For this review, take the finished solid that the model builds, in its own axes (mm). A direction names the side the tool comes from. Give positions to 0.01 mm unless a question says otherwise; leave off trailing zeros. Write each loop counter-clockwise with the first axis right and the second up, starting at its lowest first coordinate (ties: lowest second). Pieces come first, ordered by that corner, then holes. Notation, with made-up numbers: (12.25, 76.25) -> (44.25, 76.25) arc R14 cw to (44.25, 103.25) -> close; hole circle Ø7 at (-34.75, 7). An arc over 180 degrees is marked (long way). Answer as CSV lines item,"result".
```python
from build123d import *

# Parameters (mm, degrees)
BOX001_W           = 93.5
BOX001_H           = 21.5
BOX001_DEPTH       = 20.75
BOX015001015_W     = 96.5
BOX015001015_H     = 24.5
BOX015001015_DEPTH = 22.25


with BuildPart() as cube016:
    # Box001 → Box001 (new body)
    with BuildSketch(Plane(origin=(1.5, 1.5, 1.5), x_dir=(1, 0, 0), z_dir=(0, 0, 1))):
        with Locations((46.75, 10.75)):
            Rectangle(BOX001_W, BOX001_H)
    extrude(amount=BOX001_DEPTH)


with BuildPart() as cut004014:
    # Box015001015 → Box015001015 (new body)
    with BuildSketch(Plane.XY):
        with Locations((48.25, 12.25)):
            Rectangle(BOX015001015_W, BOX015001015_H)
    extrude(amount=BOX015001015_DEPTH)

    # Cut004014: cut Cube016
    add(cube016.part, mode=Mode.SUBTRACT)


with BuildPart() as cut004014_1:
    # Cut004014 placement: moved
    add(cut004014.part.moved(Location((3, -4, 0))))


solid = cut004014_1.part
```
Q1. Clearance check with a flat-ended pin moving along its axis: pin 1 (6.5 mm diameter, centred on x = 40, y = 12, fed in from +Z). State where the tip first meets the part, or that it passes through.
Answer block:
pin 1,"stops at z = 1.5"
Q2. Add section C-C (x = 44.5). Write out the cut boundary in (y, z), plus the area to 3 significant figures.
Answer block:
outline,"(-4, 0) -> (20.5, 0) -> (20.5, 22.25) -> (19, 22.25) -> (19, 1.5) -> (-2.5, 1.5) -> (-2.5, 22.25) -> (-4, 22.25) -> close"
area,"99.0 mm2"
Q3. To check wall thickness, follow probe 1 along X at (y, z) = (16, 1.75); probe 2 along Y at (x, z) = (63.5, 17.5); probe 3 along Z at (x, y) = (35.5, -2.25). State the ranges of each line that lie inside material, in increasing order. Write a range as [from, to].
Answer block:
probe 1,"x = [3, 4.5], [98, 99.5]"
probe 2,"y = [-4, -2.5], [19, 20.5]"
probe 3,"z = [0, 1.5]"
Q4. For faces 4 (the flat face through (51, 8, 1.5)), 5 (the flat face through (99.5, 8, 11)), list the 3-axis set-ups (+Z, -Z, +X, -X, +Y, -Y) from which the entire face can be reached by the end or side of a thin tool; tool diameter is ignored.
Answer block:
face 4,"+Z"
face 5,"+Z, -Z, +X, +Y, -Y"
Q5. Draft analysis for pull direction X (two halves, no side actions). For faces 1 (the flat face through (3, 8, 11)), 2 (the flat face through (51, 8, 0)), 3 (the flat face through (51, 19, 12)), state which applies: released by +X, released by -X, zero draft, split by the parting line, or undercut.
Answer block:
face 1,"released by -X"
face 2,"zero draft"
face 3,"undercut"
Q6. Add section A-A (z = 8.5). Write out the cut boundary in (x, y).
Answer block:
outline,"(3, -4) -> (99.5, -4) -> (99.5, 20.5) -> (3, 20.5) -> close; hole (4.5, -2.5) -> (98, -2.5) -> (98, 19) -> (4.5, 19) -> close"
Q7. Add section B-B (y = 8.5). Write out the cut boundary in (x, z).
Answer block:
outline,"(3, 0) -> (99.5, 0) -> (99.5, 22.25) -> (98, 22.25) -> (98, 1.5) -> (4.5, 1.5) -> (4.5, 22.25) -> (3, 22.25) -> close"
